from build123d import *

# Parameters (mm, degrees)
F1_DEPTH = 2.5


with BuildPart() as f1:
    # F0 (on Top) → F1 (new body)
    with BuildSketch(Plane.XY):
        with BuildLine():
            Line((40, -10), (40, 10))
            Line((40, 10), (20, 10))
            ThreePointArc((20, 10), (19.23682, 8.26318), (17.5, 7.5))
            ThreePointArc((17.5, 7.5), (17.388608, 7.497625), (17.277216, 7.5))
            Line((17.277216, 7.5), (-17.277216, 7.5))
            ThreePointArc((-17.277216, 7.5), (-17.388608, 7.497625), (-17.5, 7.5))
            ThreePointArc((-17.5, 7.5), (-19.23682, 8.26318), (-20, 10))
            Line((-20, 10), (-40, 10))
            Line((-40, 10), (-40, -10))
            Line((-40, -10), (-20, -10))
            ThreePointArc((-20, -10), (-19.23682, -8.26318), (-17.5, -7.5))
            ThreePointArc((-17.5, -7.5), (-17.388608, -7.497625), (-17.277216, -7.5))
            Line((-17.277216, -7.5), (17.277216, -7.5))
            ThreePointArc((17.277216, -7.5), (17.388608, -7.497625), (17.5, -7.5))
            ThreePointArc((17.5, -7.5), (19.23682, -8.26318), (20, -10))
            Line((20, -10), (40, -10))
        make_face()
    extrude(amount=F1_DEPTH)


solid = f1.part
Can you work these out from the model? Positions are in its coordinate system, mm. A direction names the side the tool comes from. Coordinates: 2 decimals unless noted, no trailing zeros. Loops run counter-clockwise (first coordinate to the right, second up) from the corner with the lowest first, then second, coordinate; pieces in that order, holes last. Notation, with made-up numbers: (33.5, 5) - (75.5, 5) arc R15 cw to (75.5, 28) - close; hole circle Ø11 at (74.5, 81.5). An arc over 180 degrees is marked (long way). Put each result on its own line as item: value. Start each with the question number.
Item 1: If we mould it in two halves opening along X, with no side actions, what happens to faces 4 (the face through (19.256, 8.282, 1.232)), 5 (the face through (0, 7.5, 1)), 6 (the face through (30, -10, 1)), 7 (the face through (-40, 0, 1))? For each: +X half, -X half, draft (parallel to the pull), parting line (faces both ways), or undercut.
Item 2: Which directions (+Z, -Z, +X, -X, +Y, -Y) give clear straight access to the entire face, cutting with the end or side of a thin tool? Please do faces 1 (the face through (-30, 10, 1)), 2 (the face through (19.218, -8.244, 1.232)), 3 (the face through (-19.218, 8.244, 1.232)).
Item 3: If I drill on line 1 along Y through (x, z) = (-17, 0.7); line 2 along X through (y, z) = (-8.25, 2.2); line 3 along X through (y, z) = (-8.5, 1.45), over which ranges is the centre line in solid material (lowest first)?
Item 4: Suppose I cut it at B-B (x = 10). Please give me the cut outline in (y, z).
Item 5: Suppose I cut it at A-A (z = 1.85). Please give me the cut outline in (x, y).
Item 6: Suppose I cut it at C-C (x = -19). Please give me the cut outline in (y, z), and give its area (3 significant figures).
Item 7: For pin 1 (0.8 mm diameter, centred on x = -2.5, z = 1, fed in from +Y); pin 2 (1.2 mm diameter, centred on x = -4.5, z = 1, fed in from -Y); pin 3 (4 mm diameter, centred on x = 11.5, y = 1.5, fed in from -Z), each with a flat end and sliding along its axis, tell me the tip position at first contact or that it passes through.
Here are the results:
1. face 4: undercut
1. face 5: undercut
1. face 6: draft
1. face 7: -X half
2. face 1: +Z, -Z, +X, -X, +Y
2. face 2: +Z, -Z, -Y
2. face 3: +Z, -Z, +Y
3. line 1: -7.5 to 7.5
3. line 2: -40 to -19.22, 19.22 to 40
3. line 3: -40 to -19.45, 19.45 to 40
4. outline: (-7.5, 0) - (7.5, 0) - (7.5, 2.5) - (-7.5, 2.5) - close
5. outline: (-40, -10) - (-20, -10) arc R2.61 cw to (-17.5, -7.5) arc R2.61 cw to (-17.28, -7.5) - (17.28, -7.5) arc R2.61 cw to (17.5, -7.5) arc R2.61 cw to (20, -10) - (40, -10) - (40, 10) - (20, 10) arc R2.61 cw to (17.5, 7.5) arc R2.61 cw to (17.28, 7.5) - (-17.28, 7.5) arc R2.61 cw to (-17.5, 7.5) arc R2.61 cw to (-20, 10) - (-40, 10) - close
6. outline: (-8.05, 0) - (8.05, 0) - (8.05, 2.5) - (-8.05, 2.5) - close
6. area: 40.3 mm²
7. pin 1: y = 7.5
7. pin 2: y = -7.5
7. pin 3: z = 0
